Can you work these out from the model? Positions are in its coordinate system, mm. A direction names the side the tool comes from. Round coordinates to 2 decimals unless told otherwise and drop trailing zeros. Loops run counter-clockwise (first coordinate to the right, second up) from the corner with the lowest first, then second, coordinate; pieces in that order, holes last. Notation, with made-up numbers: M 67.5,79 L 85.5,79 A20 ccw 85.5,94 Z; hole C 4,49 d2. An arc over 180 degrees is marked long. Return JSON: item names as keys, results as strings.
```python
from build123d import *

# Parameters (mm, degrees)
SKETCH_1_R          = 3
SKETCH_1_R_2        = 2.5
EXTRUDE_1_DEPTH     = 3
EXTRUDE_START       = -2
SKETCH_3_R          = 2.5
EXTRUDE_3_DEPTH     = 2
SKETCH_7_R          = 2.65
CUT_EXTRUDE_1_DEPTH = 1
CHAMFER_1_SIZE      = 1
CUT_EXTRUDE_3_REACH = 53.614
SKETCH_10_R         = 2.5
CUT_EXTRUDE_4_REACH = 53.662
CHAMFER_2_SIZE      = 1.5
CUT_EXTRUDE_5_REACH = 53.662
CHAMFER_3_SIZE      = 2


with BuildPart() as part:
    # 스케치1 → 보스-돌출1 (new body)
    with BuildSketch(Plane.XY):
        with BuildLine():
            Line((-27.349187557, -28.196867314), (-7.694270353, -28.196867314))
            Line((-7.694270353, -28.196867314), (-3.192250131, -23.196867314))
            Line((-3.192250131, -23.196867314), (12.267749869, -23.196867314))
            Line((12.267749869, -23.196867314), (17.250812443, -27.683637009))
            Line((17.250812443, -27.683637009), (17.250812443, -14.696867314))
            ThreePointArc((17.250812443, -14.696867314), (22.450812443, -9.496867314), (27.650812443, -14.696867314))
            Line((27.650812443, -14.696867314), (27.650812443, -28.196867314))
            Line((27.650812443, -28.196867314), (40.650812443, -28.196867314))
            Line((40.650812443, -28.196867314), (40.650812443, 12.183132686))
            Line((40.650812443, 12.183132686), (28.992507116, 23.803132686))
            Line((28.992507116, 23.803132686), (13.742507116, 23.803132686))
            Line((13.742507116, 23.803132686), (8.450812443, 28.403132686))
            Line((8.450812443, 28.403132686), (-0.749187557, 28.403132686))
            Line((-0.749187557, 28.403132686), (-5.349187557, 23.803132686))
            Line((-5.349187557, 23.803132686), (-28.149187557, 23.803132686))
            Line((-28.149187557, 23.803132686), (-43.049187557, 8.903132686))
            Line((-43.049187557, 8.903132686), (-43.049187557, -28.196867314))
            Line((-43.049187557, -28.196867314), (-37.749187557, -28.196867314))
            Line((-37.749187557, -28.196867314), (-37.749187557, -3.196867314))
            ThreePointArc((-37.749187557, -3.196867314), (-29.949187557, 1.306464785), (-29.949187557, -7.700199414))
            Line((-29.949187557, -7.700199414), (-29.949187557, -28.196867314))
            Line((-29.949187557, -28.196867314), (-27.349187557, -28.196867314))
        make_face()
        with Locations((8.802507116, -1.986867314)):
            Circle(SKETCH_1_R, mode=Mode.SUBTRACT)
        with Locations((-21.197492884, 7.013132686)):
            Circle(SKETCH_1_R_2, mode=Mode.SUBTRACT)
        with Locations((3.302507116, 22.513132686)):
            Circle(SKETCH_1_R_2, mode=Mode.SUBTRACT)
    extrude(amount=EXTRUDE_1_DEPTH)

    # 스케치3 → 보스-돌출3 (add)
    # profile 1 of 2: a face of its own
    with BuildSketch(Plane.XY.offset(3).offset(EXTRUDE_START)):
        with BuildLine():
            Line((27.650812443, -14.696867314), (27.650812443, -28.196867314))
            Line((27.650812443, -28.196867314), (17.764042748, -28.196867314))
            Line((17.764042748, -28.196867314), (17.250812443, -27.683637009))
            Line((17.250812443, -27.683637009), (17.250812443, -14.696867314))
            ThreePointArc((17.250812443, -14.696867314), (22.450812443, -9.496867314), (27.650812443, -14.696867314))
        make_face()
        with Locations((22.450812443, -14.696867314)):
            Circle(SKETCH_3_R, mode=Mode.SUBTRACT)
    # profile 2 of 2: a face of its own
    with BuildSketch(Plane.XY.offset(3).offset(EXTRUDE_START)):
        with BuildLine():
            Line((-29.949187557, -7.700199414), (-29.949187557, -28.196867314))
            Line((-29.949187557, -28.196867314), (-30.049187557, -28.196867314))
            Line((-30.049187557, -28.196867314), (-37.749187557, -28.196867314))
            Line((-37.749187557, -28.196867314), (-37.749187557, -3.196867314))
            ThreePointArc((-37.749187557, -3.196867314), (-29.949187557, 1.306464785), (-29.949187557, -7.700199414))
        make_face()
        with Locations((-32.549187557, -3.196867314)):
            Circle(SKETCH_3_R, mode=Mode.SUBTRACT)
    extrude(amount=EXTRUDE_3_DEPTH)

    # 스케치7 → 컷-돌출1 (cut)
    with BuildSketch(Plane(origin=(0, 0, 0), x_dir=(-1, 0, 0), z_dir=(0, 0, -1))):
        with Locations((6.149187557, 20.803132686)):
            Circle(SKETCH_7_R)
        with Locations((8.049187557, -24.196867314)):
            Circle(SKETCH_7_R)
        with BuildLine():
            Line((-26.406412787, 7.908733029), (-32.895212099, 7.908733029))
            ThreePointArc((-32.895212099, 7.908733029), (-33.708384897, 8.245560231), (-34.045212099, 9.058733029))
            Line((-34.045212099, 9.058733029), (-34.045212099, 15.547532342))
            ThreePointArc((-34.045212099, 15.547532342), (-33.708384897, 16.36070514), (-32.895212099, 16.697532342))
            Line((-32.895212099, 16.697532342), (-29.650812443, 16.697532342))
            ThreePointArc((-29.650812443, 16.697532342), (-26.543502647, 15.410442482), (-25.256412787, 12.303132686))
            Line((-25.256412787, 12.303132686), (-25.256412787, 9.058733029))
            ThreePointArc((-25.256412787, 9.058733029), (-25.593239988, 8.245560231), (-26.406412787, 7.908733029))
        make_face()
    extrude(amount=-CUT_EXTRUDE_1_DEPTH, mode=Mode.SUBTRACT)

    # 모따기1
    chamfer_1_edges = [part.edges().sort_by_distance(p)[0] for p in [
        (-43.049187557, -28.196867314, 1.5),
        (40.650812443, -28.196867314, 1.5),
    ]]
    chamfer(chamfer_1_edges, length=CHAMFER_1_SIZE)

    # 스케치10 → 컷-돌출3 (cut, up to next)
    with BuildSketch(Plane(origin=(0, 0, 1), x_dir=(-1, 0, 0), z_dir=(0, 0, -1)), mode=Mode.PRIVATE) as cut_extrude_3_sk1:
        with Locations((-29.650812443, 12.303132686)):
            Circle(SKETCH_10_R)
    cut_extrude_3_tool1 = extrude(cut_extrude_3_sk1.sketch, amount=-CUT_EXTRUDE_3_REACH, mode=Mode.PRIVATE) & part.part
    add(cut_extrude_3_tool1.solids().sort_by_distance((29.650812, 12.303133, 1))[0], mode=Mode.SUBTRACT)

    # 스케치12 → 컷-돌출4 (cut, up to next)
    with BuildSketch(Plane(origin=(0, 0, 0), x_dir=(-1, 0, 0), z_dir=(0, 0, -1)), mode=Mode.PRIVATE) as cut_extrude_4_sk1:
        Polygon((16.749187557, 23.803132686), (16.749187557, 16.353132686), (35.599187557, 16.353132686), (28.149187557, 23.803132686), align=None)
    cut_extrude_4_tool1 = extrude(cut_extrude_4_sk1.sketch, amount=-CUT_EXTRUDE_4_REACH, mode=Mode.PRIVATE) & part.part
    add(cut_extrude_4_tool1.solids().sort_by_distance((-24.464587, 19.772334, 0))[0], mode=Mode.SUBTRACT)

    # 모따기2
    chamfer_2_edges = [part.edges().sort_by_distance(p)[0] for p in [
        (-16.749187557, 23.803132686, 1.5),
        (-16.749187557, 16.353132686, 1.5),
    ]]
    chamfer(chamfer_2_edges, length=CHAMFER_2_SIZE)

    # 스케치13 → 컷-돌출5 (cut, up to next)
    with BuildSketch(Plane(origin=(0, 0, 0), x_dir=(-1, 0, 0), z_dir=(0, 0, -1)), mode=Mode.PRIVATE) as cut_extrude_5_sk1:
        Polygon((-34.689283113, 18.125074406), (-34.689283113, -28.196867314), (-39.650812443, -28.196867314), (-40.650812443, -27.196867314), (-40.650812443, 12.183132686), align=None)
    cut_extrude_5_tool1 = extrude(cut_extrude_5_sk1.sketch, amount=-CUT_EXTRUDE_5_REACH, mode=Mode.PRIVATE) & part.part
    # 스케치13 → 컷-돌출5 (cut, up to next)
    with BuildSketch(Plane(origin=(0, 0, 0), x_dir=(-1, 0, 0), z_dir=(0, 0, -1)), mode=Mode.PRIVATE) as cut_extrude_5_sk2:
        Polygon((38.049187557, 13.903132686), (43.049187557, 8.903132686), (43.049187557, -27.196867314), (42.049187557, -28.196867314), (38.049187557, -28.196867314), align=None)
    cut_extrude_5_tool2 = extrude(cut_extrude_5_sk2.sketch, amount=-CUT_EXTRUDE_5_REACH, mode=Mode.PRIVATE) & part.part
    add(cut_extrude_5_tool1.solids().sort_by_distance((37.59669, -6.446011, 0))[0], mode=Mode.SUBTRACT)
    add(cut_extrude_5_tool2.solids().sort_by_distance((-40.49096, -8.321213, 0))[0], mode=Mode.SUBTRACT)

    # 모따기3
    chamfer_3_edges = [part.edges().sort_by_distance(p)[0] for p in [
        (-38.049187557, -28.196867314, 1.5),
        (34.689283113, -28.196867314, 1.5),
    ]]
    chamfer(chamfer_3_edges, length=CHAMFER_3_SIZE)


solid = part.part
```
Q1. Thinking about a two-plate mould opening in Y: for faces 1 (the cylindrical face through (-23.04, 8.7, 1.48)), 2 (the flat face through (25, -28.197, 2)), 3 (the flat face through (-16.749, 20, 1)), which applies, pulls with the +Y half, pulls with the -Y half, needs draft (parallel to the pull), parting line crosses it, or undercut?
Results:
{"face 1": "undercut", "face 2": "pulls with the -Y half", "face 3": "needs draft"}
Q2. I'm going to push flat-ended pins straight in: pin 1 Ø4.5 at (x, y) = (29.65, 12.3) entering from +Z; pin 2 Ø9.5 at (x, y) = (-32.55, -3.2) entering from +Z; pin 3 Ø6.5 at (x, y) = (-32.55, -3.2) entering from -Z. Where does each tip first touch, or does it pass through?
Results:
{"pin 1": "passes through", "pin 2": "stops at z = 3", "pin 3": "stops at z = 1"}
Q3. Suppose I cut it at C-C, the plane z = 2.45. Please give me the cut outline in (x, y).
Results:
{"outline": "M -38.05,-26.2 L -36.05,-28.2 L -7.69,-28.2 L -3.19,-23.2 L 12.27,-23.2 L 17.25,-27.68 L 17.76,-28.2 L 32.69,-28.2 L 34.69,-26.2 L 34.69,18.13 L 28.99,23.8 L 13.74,23.8 L 8.45,28.4 L -0.75,28.4 L -5.35,23.8 L -15.25,23.8 L -16.75,22.3 L -16.75,17.85 L -18.25,16.35 L -35.6,16.35 L -38.05,13.9 Z; hole C -32.55,-3.2 d5; hole C -21.2,7.01 d5; hole C 3.3,22.51 d5; hole C 8.8,-1.99 d6; hole C 22.45,-14.7 d5; hole C 29.65,12.3 d5"}
Q4. Suppose I cut it at A-A, the plane x = 3.5. Please give me the cut outline in (y, z).
Results:
{"outline": "M -23.2,0 L 20.02,0 L 20.02,3 L -23.2,3 Z; M 25.01,0 L 28.4,0 L 28.4,3 L 25.01,3 Z"}
Q5. If I drill on line 1 along Y through (x, z) = (3.5, 1.95); line 2 along X through (y, z) = (-2, 2.55); line 3 along X through (y, z) = (10, 0.9), over which ranges is the centre line in solid material (lowest first)?
Results:
{"line 1": "y = -23.2 to 20.02, 25.01 to 28.4", "line 2": "x = -38.05 to -34.74, -30.35 to 5.8, 11.8 to 34.69", "line 3": "x = -38.05 to 25.26, 34.05 to 34.69"}
Q6. Suppose I cut it at D-D, the plane x = 22. Please give me the cut outline in (y, z).
Results:
{"outline": "M -28.2,1 L -17.16,1 L -17.16,3 L -28.2,3 Z; M -12.24,1 L -9.52,1 L -9.52,0 L 23.8,0 L 23.8,3 L -12.24,3 Z"}
Q7. On a 3-axis mill with a long thin cutter (end or side, diameter ignored), from which of +Z, -Z, +X, -X, +Y, -Y can I reach the whole of each face in a straight line? I mean faces 4 (the flat face through (21, 23.803, 1)), 5 (the flat face through (32, 10, 1)), 6 (the flat face through (-5.475, -25.732, 1.479)), 7 (the flat face through (-10, 23.803, 1)). Say none if no direction works.
Results:
{"face 4": "+Z, -Z, +X, +Y", "face 5": "-Z", "face 6": "+Z, -Z, -Y", "face 7": "+Z, -Z, -X, +Y"}
Q8. Suppose I cut it at B-B, the plane y = -13.5. Please give me the cut outline in (x, z), plus the area to 3 significant figures.
Results:
{"outline": "M -38.05,0 L -37.75,0 L -37.75,1 L -29.95,1 L -29.95,0 L 17.39,0 L 17.39,1 L 20.26,1 L 20.26,3 L -38.05,3 Z; M 24.65,1 L 27.51,1 L 27.51,0 L 34.69,0 L 34.69,3 L 24.65,3 Z", "area": "192 mm2"}
